from build123d import *

# Parameters (mm, degrees)
BOSS_EXTRUDE1_START = 3
BOSS_EXTRUDE1_DEPTH = 1
BOSS_EXTRUDE2_START = 0.5
SKETCH1_3_R         = 2
BOSS_EXTRUDE2_DEPTH = 3.5
FILLET1_R           = 10
SKETCH2_R           = 3.5
CUT_EXTRUDE1_DEPTH  = 2


with BuildPart() as part:
    # Sketch1 → Boss-Extrude1 (new body)
    with BuildSketch(Plane.XY.offset(BOSS_EXTRUDE1_START)):
        Polygon((-103.211042913, -22.2), (-31.211042913, -22.2), (-31.211042913, 36.8), (-90.311042913, 36.8), (-90.311042913, 32.8), (-99.211042913, 32.8), (-99.211042913, 36.8), (-103.211042913, 36.8), align=None)
    extrude(amount=BOSS_EXTRUDE1_DEPTH)

    # Sketch1<3> → Boss-Extrude2 (add)
    # profile 1 of 2: a face of its own
    with BuildSketch(Plane.XY.offset(BOSS_EXTRUDE2_START)):
        with BuildLine():
            Line((-108.511042913, 1.8), (-103.211042913, 1.8))
            Line((-103.211042913, 1.8), (-103.211042913, 12.8))
            Line((-103.211042913, 12.8), (-108.511042913, 12.8))
            ThreePointArc((-108.511042913, 12.8), (-114.011042913, 7.3), (-108.511042913, 1.8))
        make_face()
        with Locations((-108.711042913, 7.3)):
            Circle(SKETCH1_3_R, mode=Mode.SUBTRACT)
    # profile 2 of 2: a face of its own
    with BuildSketch(Plane.XY.offset(BOSS_EXTRUDE2_START)):
        with BuildLine():
            Line((-31.211042913, 12.8), (-31.211042913, 1.8))
            Line((-31.211042913, 1.8), (-25.911042913, 1.8))
            ThreePointArc((-25.911042913, 1.8), (-20.411042913, 7.3), (-25.911042913, 12.8))
            Line((-25.911042913, 12.8), (-31.211042913, 12.8))
        make_face()
        with Locations((-25.711042913, 7.3)):
            Circle(SKETCH1_3_R, mode=Mode.SUBTRACT)
    extrude(amount=BOSS_EXTRUDE2_DEPTH)

    # Fillet1
    # the kernel refuses this fillet: 10 mm, written as the material it adds along each edge
    with BuildSketch(Plane(origin=(-31.211042913, 1.8, 3), x_dir=(-1, 0, 0), z_dir=(0, 1, 0)), Plane(origin=(-103.211042913, 12.8, 3), x_dir=(1, 0, 0), z_dir=(0, -1, 0))) as fillet1_piece_1:
        with BuildLine():
            CenterArc((6.614378278, -10), FILLET1_R, 90, 41.409622109)
            Line((0, -2.5), (0, 0))
            Line((0, 0), (6.614378278, 0))
        make_face()
    extrude(amount=11)

    # Sketch2 → Cut-Extrude1 (cut)
    with BuildSketch(Plane.XY.offset(4)):
        with Locations((-108.711042913, 7.3)):
            Circle(SKETCH2_R)
        with Locations((-25.711042913, 7.3)):
            Circle(SKETCH2_R)
    extrude(amount=-CUT_EXTRUDE1_DEPTH, mode=Mode.SUBTRACT)


solid = part.part
Here's how the part is built. I have some questions about the finished solid (model axes, mm). A direction names the side the tool comes from. Coordinates: 2 decimals unless noted, no trailing zeros. Loops run counter-clockwise (first coordinate to the right, second up) from the corner with the lowest first, then second, coordinate; pieces in that order, holes last. Notation, with made-up numbers: (17, -25.75) -> (71, -25.75) arc R21 cw to (71, 6.25) -> close; hole circle Ø1 at (-11.75, -18.5). An arc over 180 degrees is marked (long way). Use one line per item in the form item = value. Start each with the question number.
(1) We'd pull the mould along Y, two halves only. Please class faces 4 (the face through (-26, 5, 2)), 5 (the face through (-68, 8, 4)), 6 (the face through (-20.412, 7.179, 2.226)): pulls with the +Y half, pulls with the -Y half, needs draft (parallel to the pull), parting line crosses it, or undercut.
(2) Will these pins go through, and if not, where does the flat tip stop? pin 1 (1.1 mm diameter, centred on y = -7, z = 3.5, fed in from +X); pin 2 (1.1 mm diameter, centred on x = -94, z = 3.5, fed in from +Y); pin 3 (3 mm diameter, centred on x = -108.71, y = 7.3, fed in from -Z); pin 4 (1.1 mm diameter, centred on y = -6, z = 3.5, fed in from -X).
(3) Please list where these lines run through material, in increasing order: line 1 along X through (y, z) = (7.3, 0.85); line 2 along X through (y, z) = (7.3, 0.8); line 3 along Y through (x, z) = (-31, 1.5).
(4) If we section it at B-B (x = -35.5): Please give me the cut outline in (y, z), then the cut area to 3 significant figures.
(5) If we section it at C-C (y = -1): Please give me the cut outline in (x, z), then the cut area to 3 significant figures.
(6) If we section it at A-A (y = 7.3): Please give me the cut outline in (x, z).
(7) On a 3-axis mill with a long thin cutter (end or side, diameter ignored), from which of +Z, -Z, +X, -X, +Y, -Y can I reach the whole of each face in a straight line? I mean faces 1 (the face through (-114.01, 7.42, 2.23)), 2 (the face through (-100.085, 7.377, 2.372)), 3 (the face through (-29.208, 7.454, 3.014)). Say none if no direction works.
(8) If we section it at D-D (x = -49): Please give me the cut outline in (y, z).
Verdict:
q1.face_4 = undercut
q1.face_5 = needs draft
q1.face_6 = parting line crosses it
q2.pin_1 = -31.21
q2.pin_2 = 32.8
q2.pin_3 = through
q2.pin_4 = -103.21
q3.line_1 = -114.01 to -110.71, -106.71 to -102.79, -31.63 to -27.71, -23.71 to -20.41
q3.line_2 = -114.01 to -110.71, -106.71 to -102.85, -31.57 to -27.71, -23.71 to -20.41
q3.line_3 = 1.8 to 12.8
q4.outline = (-22.2, 3) -> (1.8, 3) -> (1.8, 2.73) -> (12.8, 2.73) -> (12.8, 3) -> (36.8, 3) -> (36.8, 4) -> (-22.2, 4) -> close
q4.area = 62.0 mm²
q5.outline = (-103.21, 3) -> (-31.21, 3) -> (-31.21, 4) -> (-103.21, 4) -> close
q5.area = 72.0 mm²
q6.outline = (-114.01, 0.5) -> (-110.71, 0.5) -> (-110.71, 2) -> (-112.21, 2) -> (-112.21, 4) -> (-114.01, 4) -> close; (-106.71, 0.5) -> (-103.21, 0.5) arc R10 cw to (-96.6, 3) -> (-37.83, 3) arc R10 cw to (-31.21, 0.5) -> (-27.71, 0.5) -> (-27.71, 2) -> (-29.21, 2) -> (-29.21, 4) -> (-105.21, 4) -> (-105.21, 2) -> (-106.71, 2) -> close; (-23.71, 0.5) -> (-20.41, 0.5) -> (-20.41, 4) -> (-22.21, 4) -> (-22.21, 2) -> (-23.71, 2) -> close
q7.face_1 = +Z, -Z, -X
q7.face_2 = -Z, +Y, -Y
q7.face_3 = +Z
q8.outline = (-22.2, 3) -> (36.8, 3) -> (36.8, 4) -> (-22.2, 4) -> close
